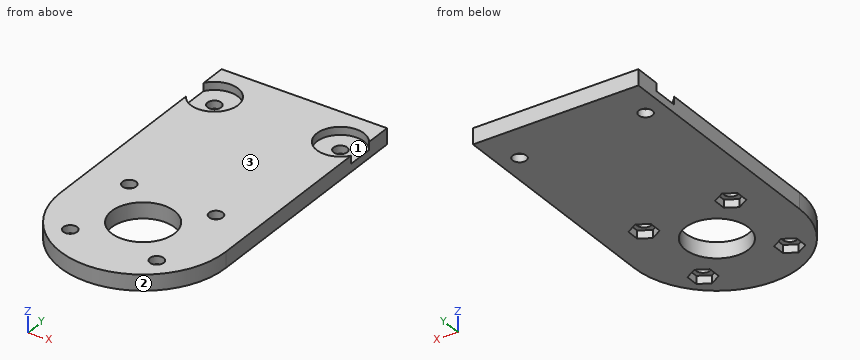
from build123d import *

# Parameters (mm, degrees)
BOSS_EXTRUDE1_DEPTH = 4
SKETCH2_R           = 6
CUT_EXTRUDE1_DEPTH  = 64.694583757
SKETCH3_R           = 8
CUT_EXTRUDE2_DEPTH  = 4
SKETCH4_R           = 1.75
CUT_EXTRUDE3_DEPTH  = 64.694583757
CUT_EXTRUDE4_DEPTH  = 2
SKETCH6_R           = 1.75
CUT_EXTRUDE5_DEPTH  = 64.694583757
SKETCH7_R           = 6
CUT_EXTRUDE6_DEPTH  = 2


with BuildPart() as part:
    # Sketch1 → Boss-Extrude1 (new body)
    with BuildSketch(Plane.XY):
        with BuildLine():
            Line((-21, 0), (-21, 60))
            Line((-21, 60), (21, 60))
            Line((21, 60), (21, 0))
            ThreePointArc((21, 0), (0, -21), (-21, 0))
        make_face()
    extrude(amount=BOSS_EXTRUDE1_DEPTH)

    # Sketch2 → Cut-Extrude1 (cut, through all)
    with BuildSketch(Plane(origin=(0, 0, 0), x_dir=(-1, 0, 0), z_dir=(0, 0, -1))):
        Circle(SKETCH2_R)
    extrude(amount=-CUT_EXTRUDE1_DEPTH, mode=Mode.SUBTRACT)

    # Sketch3 → Cut-Extrude2 (cut)
    with BuildSketch(Plane(origin=(0, 0, 0), x_dir=(-1, 0, 0), z_dir=(0, 0, -1))):
        Circle(SKETCH3_R)
    extrude(amount=-CUT_EXTRUDE2_DEPTH, mode=Mode.SUBTRACT)

    # Sketch4 → Cut-Extrude3 (cut, through all)
    with BuildSketch(Plane(origin=(0, 0, 0), x_dir=(-1, 0, 0), z_dir=(0, 0, -1))):
        with Locations((-11, -11)):
            Circle(SKETCH4_R)
        with Locations(Location((-11, 11, 0), (0, 0, 180))):
            Circle(SKETCH4_R)
        with Locations((11, 11)):
            Circle(SKETCH4_R)
        with Locations(Location((11, -11, 0), (0, 0, 180))):
            Circle(SKETCH4_R)
    extrude(amount=-CUT_EXTRUDE3_DEPTH, mode=Mode.SUBTRACT)

    # Sketch5 → Cut-Extrude4 (cut)
    with BuildSketch(Plane(origin=(0, 0, 0), x_dir=(-1, 0, 0), z_dir=(0, 0, -1))):
        Polygon((-11, -7.709103466), (-13.85, -9.354551733), (-13.85, -12.645448267), (-11, -14.290896534), (-8.15, -12.645448267), (-8.15, -9.354551733), align=None)
        Polygon((-8.15, 9.354551733), (-11, 7.709103466), (-13.85, 9.354551733), (-13.85, 12.645448267), (-11, 14.290896534), (-8.15, 12.645448267), align=None)
        Polygon((11, 7.709103466), (13.85, 9.354551733), (13.85, 12.645448267), (11, 14.290896534), (8.15, 12.645448267), (8.15, 9.354551733), align=None)
        Polygon((8.15, -9.354551733), (11, -7.709103466), (13.85, -9.354551733), (13.85, -12.645448267), (11, -14.290896534), (8.15, -12.645448267), align=None)
    extrude(amount=-CUT_EXTRUDE4_DEPTH, mode=Mode.SUBTRACT)

    # Sketch6 → Cut-Extrude5 (cut, through all)
    with BuildSketch(Plane(origin=(0, 0, 0), x_dir=(-1, 0, 0), z_dir=(0, 0, -1))):
        with Locations((-16, 50)):
            Circle(SKETCH6_R)
        with Locations(Location((16, 50, 0), (0, 0, 180))):
            Circle(SKETCH6_R)
    extrude(amount=-CUT_EXTRUDE5_DEPTH, mode=Mode.SUBTRACT)

    # Sketch7 → Cut-Extrude6 (cut)
    with BuildSketch(Plane.XY.offset(4)):
        with Locations((-16, 50)):
            Circle(SKETCH7_R)
        with Locations((16, 50)):
            Circle(SKETCH7_R)
    extrude(amount=-CUT_EXTRUDE6_DEPTH, mode=Mode.SUBTRACT)


solid = part.part
For this review, take the finished solid that the model builds, in its own axes (mm). Face numbers are marked on the shaded views. Round coordinates to 2 decimals unless told otherwise and drop trailing zeros. Order: outer loops, then holes, each group sorted by start corner. A loop starts at its lowest first (then second) coordinate and runs counter-clockwise, first axis right, second up. Notation, with made-up numbers: (-16.75, 46.25) -> (38.25, 46.25) arc R13 ccw to (38.25, 56.25) -> close; hole circle Ø5 at (10, 36.5). An arc over 180 degrees is marked (long way). Put each result on its own line as item: value.
Q1. Mouldability with a two-part tool opening along X and no side actions: class the marked faces 1, 2 and 3 as pulls with the +X half, pulls with the -X half, needs draft (parallel to the pull), parting line crosses it, or undercut.
Check result:
face 1: undercut
face 2: parting line crosses it
face 3: needs draft
Q2. Insertion check: pin 1 Ø2 at (x, y) = (-16, 50) entering from +Z; pin 2 Ø4.5 at (x, y) = (16, 50) entering from +Z; pin 3 Ø4 at (x, y) = (-11, -11) entering from -Z; pin 4 Ø1.6 at (y, z) = (-11, 1) entering from -X. Each pin has a flat end and moves straight along its axis. Give the tip position at first contact, or say it passes through.
Check result:
pin 1: through
pin 2: z = 2
pin 3: z = 2
pin 4: x = -18.36
Q3. Add section A-A on x = 0. Write out the cut boundary in (y, z).
Check result:
outline: (-21, 0) -> (-8, 0) -> (-8, 4) -> (-21, 4) -> close; (8, 0) -> (60, 0) -> (60, 4) -> (8, 4) -> close
Q4. Add section C-C on z = 3.1. Write out the cut boundary in (x, y).
Check result:
outline: (-21, 0) arc R21 ccw to (21, 0) -> (21, 46.68) arc R6 cw (long way) to (21, 53.32) -> (21, 60) -> (-21, 60) -> (-21, 53.32) arc R6 cw (long way) to (-21, 46.68) -> close; hole circle Ø3.5 at (-11, -11); hole circle Ø3.5 at (-11, 11); hole circle Ø16 at (0, 0); hole circle Ø3.5 at (11, -11); hole circle Ø3.5 at (11, 11)
Q5. Add section B-B on y = 50. Write out the cut boundary in (x, z).
Check result:
outline: (-21, 0) -> (-17.75, 0) -> (-17.75, 2) -> (-21, 2) -> close; (-14.25, 0) -> (14.25, 0) -> (14.25, 2) -> (10, 2) -> (10, 4) -> (-10, 4) -> (-10, 2) -> (-14.25, 2) -> close; (17.75, 0) -> (21, 0) -> (21, 2) -> (17.75, 2) -> close
Q6. For probe 1 along Y at (x, z) = (-11.5, 2.25); probe 2 along Y at (x, z) = (-11, 3); probe 3 along Y at (x, z) = (11.5, 1.4), list the stretches that pass through material, from the lowest coordinate up. Write a range as [from, to].
Check result:
probe 1: [-17.57, -12.68], [-9.32, 9.32], [12.68, 46.03], [53.97, 60]
probe 2: [-17.89, -12.75], [-9.25, 9.25], [12.75, 46.68], [53.32, 60]
probe 3: [-17.57, -14], [-8, 8], [14, 60]
Q7. Add section D-D on y = 13.5. Write out the cut boundary in (x, z).
Check result:
outline: (-21, 0) -> (-12.37, 0) -> (-12.37, 2) -> (-9.63, 2) -> (-9.63, 0) -> (9.63, 0) -> (9.63, 2) -> (12.37, 2) -> (12.37, 0) -> (21, 0) -> (21, 4) -> (-21, 4) -> close
